Geometry check sheet. Reference: the model listing, model coordinates, mm. Face numbers are marked on the shaded views. A direction names the side the tool comes from. Give positions to 0.01 mm unless a question says otherwise; leave off trailing zeros. Loops run counter-clockwise (first coordinate to the right, second up) from the corner with the lowest first, then second, coordinate; pieces in that order, holes last. Notation, with made-up numbers: (4.25, 36) -> (13.25, 36) arc R30 cw to (13.25, 69) -> close; hole circle Ø6 at (41, 36.25). An arc over 180 degrees is marked (long way). One line per item, written item: value. Start each with the question number.
(1) Tool access check on the marked faces 4, 5, 6, 7 and 8. Record the directions out of +Z, -Z, +X, -X, +Y, -Y that give a thin tool (end or side, any length) a straight path to the whole face; none if there is none.
(2) Sectioned sample at D-D, the plane x = -26. Record the cut outline in (y, z).
(3) Gauge pin test, flat ends, axial feed: pin 1 Ø1 at (x, y) = (-10, 15.5) entering from +Z; pin 2 Ø8.5 at (x, z) = (-20.5, 10) entering from -Y; pin 3 Ø8.5 at (x, z) = (-21, 9) entering from +Y. Record the tip position at first contact, or that the pin passes through.
(4) Sectioned sample at A-A, the plane x = 0. Record the cut outline in (y, z), then the cut area to 3 significant figures.
(5) Scan lines: line 1 along Y through (x, z) = (0, 4); line 2 along X through (y, z) = (8.5, 30.5); line 3 along Z through (x, y) = (-23, 0). Record each from-to range of solid material in increasing order. Write a range as from..to.
(6) Sectioned sample at C-C, the plane z = 12. Record the cut outline in (x, y), then the cut area to 3 significant figures.
(7) Sectioned sample at B-B, the plane y = 0. Record the cut outline in (x, z), then the cut area to 3 significant figures.
(8) Draft check along X on the marked faces 1, 2 and 3. Enter one of: pulls with the +X half, pulls with the -X half, needs draft (parallel to the pull), parting line crosses it, or undercut.
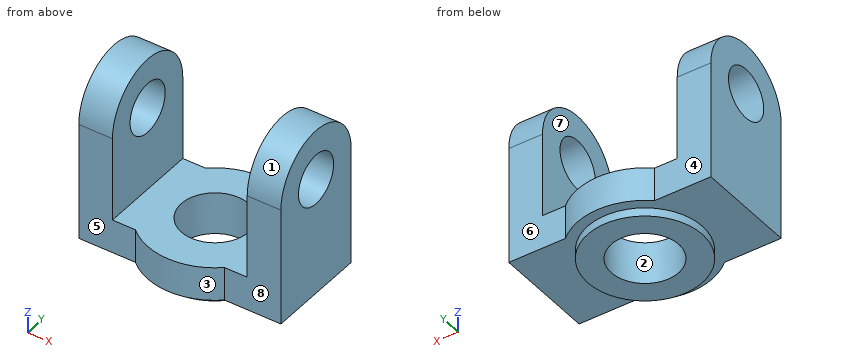
from build123d import *

# Parameters (mm, degrees)
F0_R          = 7.5
F1_DEPTH      = 30
F2_W          = 40
F2_H          = 40
F3_DEPTH      = 25
F3_DEPTH_BACK = 25
F4_R          = 20
F5_DEPTH      = 10
F6_R          = 10
F7_DEPTH      = 50.001
F7_DEPTH_BACK = 25
F8_R          = 17
F9_DEPTH      = 2.5
F10_DEPTH     = 25


with BuildPart() as f1:
    # F0 (on Right) → F1 (new body, symmetric)
    with BuildSketch(Plane.YZ):
        with BuildLine():
            Line((-15, 35), (-15, 0))
            Line((-15, 0), (15, 0))
            Line((15, 0), (15, 35))
            ThreePointArc((15, 35), (0, 50), (-15, 35))
        make_face()
        with Locations((0, 35)):
            Circle(F0_R, mode=Mode.SUBTRACT)
    extrude(amount=F1_DEPTH, both=True)

    # F2 (on Front) → F3 (cut, two sides)
    with BuildSketch(Plane.XZ) as f3_sk:
        with Locations((0, 30)):
            Rectangle(F2_W, F2_H)
    extrude(amount=-F3_DEPTH, mode=Mode.SUBTRACT)
    extrude(f3_sk.sketch, amount=F3_DEPTH_BACK, mode=Mode.SUBTRACT)

    # F4 (on Top) → F5 (join)
    with BuildSketch(Plane.XY):
        Circle(F4_R)
    extrude(amount=F5_DEPTH)

    # F6 (on Top) → F7 (cut, two sides)
    with BuildSketch(Plane.XY) as f7_sk:
        Circle(F6_R)
    extrude(amount=F7_DEPTH, mode=Mode.SUBTRACT)
    extrude(f7_sk.sketch, amount=-F7_DEPTH_BACK, mode=Mode.SUBTRACT)

    # F8 (on Top) → F9 (join)
    with BuildSketch(Plane.XY):
        Circle(F8_R)
    extrude(amount=-F9_DEPTH)

    # F10 (cut): a face of the model
    f10_faces = [f1.faces().sort_by_distance(p)[0] for p in [
        (0, 0, 0),
    ]]
    extrude(f10_faces, amount=-F10_DEPTH, mode=Mode.SUBTRACT)


solid = f1.part
Calculated:
1. face 4: +Z, -Z, -X, +Y
1. face 5: +Z, -Z, -X, -Y
1. face 6: +Z, -Z, +X, +Y
1. face 7: +Z, +Y, -Y
1. face 8: +Z, -Z, +X, -Y
2. outline: (-15, 0) -> (15, 0) -> (15, 35) arc R15 ccw to (-15, 35) -> close; hole circle Ø15 at (0, 35)
3. pin 1: stops at z = 10
3. pin 2: stops at y = -15
3. pin 3: stops at y = 15
4. outline: (-20, 0) -> (-17, 0) -> (-17, -2.5) -> (-10, -2.5) -> (-10, 10) -> (-20, 10) -> close; (10, -2.5) -> (17, -2.5) -> (17, 0) -> (20, 0) -> (20, 10) -> (10, 10) -> close
4. area: 235 mm2
5. line 1: y = -20..-10, 10..20
5. line 2: x = -30..-20, 20..30
5. line 3: z = 0..27.5, 42.5..50
6. outline: (-30, -15) -> (-20, -15) -> (-20, 15) -> (-30, 15) -> close; (20, -15) -> (30, -15) -> (30, 15) -> (20, 15) -> close
6. area: 600 mm2
7. outline: (-30, 0) -> (-17, 0) -> (-17, -2.5) -> (-10, -2.5) -> (-10, 10) -> (-20, 10) -> (-20, 27.5) -> (-30, 27.5) -> close; (-30, 42.5) -> (-20, 42.5) -> (-20, 50) -> (-30, 50) -> close; (10, -2.5) -> (17, -2.5) -> (17, 0) -> (30, 0) -> (30, 27.5) -> (20, 27.5) -> (20, 10) -> (10, 10) -> close; (20, 42.5) -> (30, 42.5) -> (30, 50) -> (20, 50) -> close
7. area: 935 mm2
8. face 1: needs draft
8. face 2: undercut
8. face 3: parting line crosses it
